Geometry: see drawing. Coordinates: mm, zero at the bounding-box minimum. Round coordinates to 2 decimals unless told otherwise and drop trailing zeros. Order: outer loops, then holes, each group sorted by start corner. A loop starts at its lowest first (then second) coordinate and runs counter-clockwise, first axis right, second up. Notation, with made-up numbers: (19.5, -27) -> (61.5, -27) arc R17 cw to (61.5, -13) -> close; hole circle Ø6 at (18.25, -18.75). An arc over 180 degrees is marked (long way). Use a Markdown table: item, result.
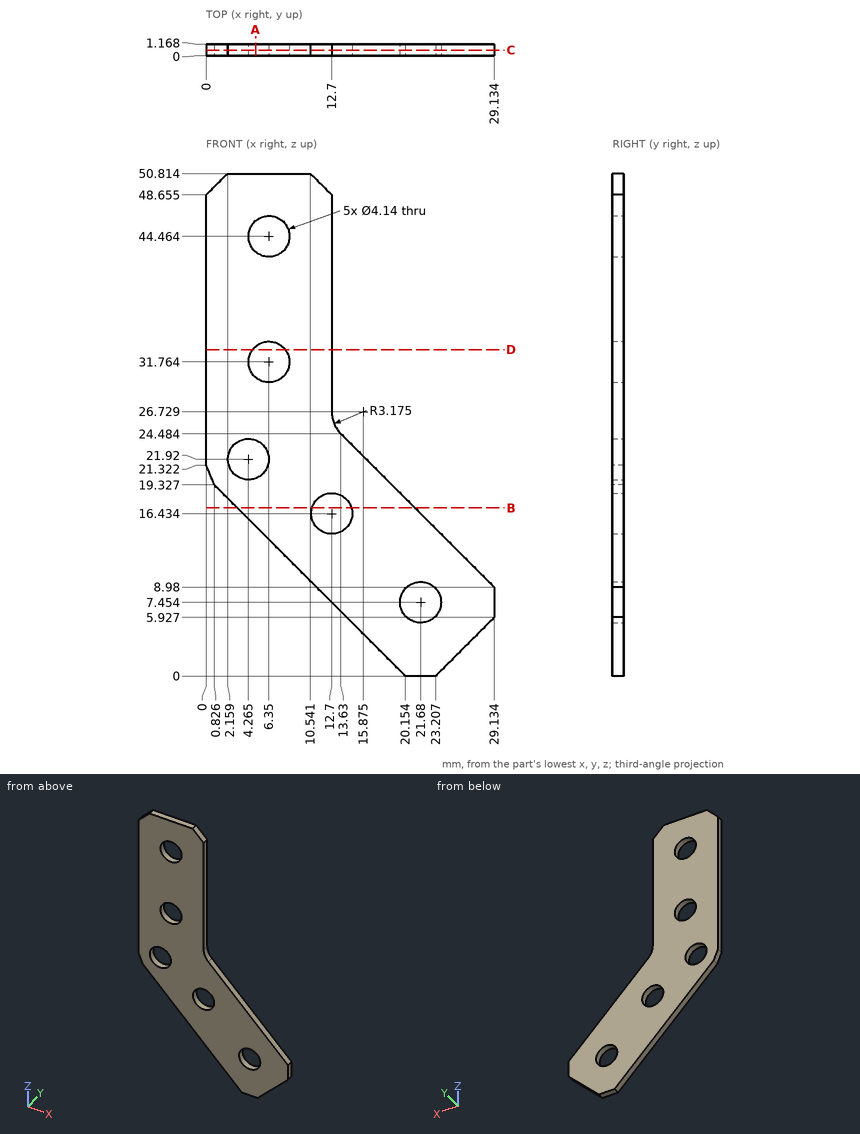
1) Cut plane C-C on y = 0.55. State how many separate pieces and enclosed holes the cut face has, and give its area (3 significant figures).
Answer key:
| item | result |
|---|---|
| separate pieces | 1 |
| enclosed holes | 5 |
| area | 635 mm^2 |
2) Cut plane B-B on z = 17. Return loops of the section in (x, y) (1 decimal).
Answer key:
| item | result |
|---|---|
| outline | (3.2, 0) -> (10.7, 0) -> (10.7, 1.2) -> (3.2, 1.2) -> close; (14.7, 0) -> (21.1, 0) -> (21.1, 1.2) -> (14.7, 1.2) -> close |
3) Cut plane A-A on x = 5. Return loops of the section in (y, z) (1 decimal).
Answer key:
| item | result |
|---|---|
| outline | (0, 15.2) -> (1.2, 15.2) -> (1.2, 20) -> (0, 20) -> close; (0, 23.9) -> (1.2, 23.9) -> (1.2, 30.2) -> (0, 30.2) -> close; (0, 33.3) -> (1.2, 33.3) -> (1.2, 42.9) -> (0, 42.9) -> close; (0, 46) -> (1.2, 46) -> (1.2, 50.8) -> (0, 50.8) -> close |
4) Ray query, probe 1 along X at (y, z) = (0.7, 36.5); probe 2 along X at (y, z) = (1, 30.5); probe 3 along X at (y, z) = (0.2, 30) (1 decimal). Return the intervals inside material, ascending.
Answer key:
| item | result |
|---|---|
| probe 1 | x = 0 to 12.7 |
| probe 2 | x = 0 to 4.71, 7.99 to 12.7 |
| probe 3 | x = 0 to 5.3, 7.4 to 12.7 |
5) Contact query for a flat-ended pin moving along its axis: P1, Ø3.5, axis at x = 6.35, z = 44.46, coming from the +Y side. Output: stop coordinate, or through.
Answer key:
| item | result |
|---|---|
| P1 | passes through |
6) Cut plane D-D on z = 33. Return loops of the section in (x, y).
Answer key:
| item | result |
|---|---|
| outline | (0, 0) -> (4.69, 0) -> (4.69, 1.17) -> (0, 1.17) -> close; (8.01, 0) -> (12.7, 0) -> (12.7, 1.17) -> (8.01, 1.17) -> close |
